```python
from build123d import *

# Parameters (mm, degrees)
ESBO_O1_W                = 170.2
ESBO_O1_H                = 111.2
RESSALTO_EXTRUS_O1_DEPTH = 0.9
ESBO_O4_W                = 176.2
ESBO_O4_H                = 117.2
RESSALTO_EXTRUS_O3_DEPTH = 1
ESBO_O5_W                = 32
ESBO_O5_H                = 1.9
CORTE_EXTRUS_O3_DEPTH    = 5
ESBO_O6_R                = 1.25
RESSALTO_EXTRUS_O4_DEPTH = 2.5
ESBO_O10_W               = 13
ESBO_O10_H               = 4
CORTE_EXTRUS_O6_DEPTH    = 1.1
ESBO_O12_W               = 146.2
ESBO_O12_H               = 82.2
CORTE_EXTRUS_O8_DEPTH    = 10


with BuildPart() as part:
    # Esboço1 → Ressalto-extrusão1 (new body)
    with BuildSketch(Plane.XY):
        with Locations((91, 62.6)):
            Rectangle(ESBO_O1_W, ESBO_O1_H)
    extrude(amount=RESSALTO_EXTRUS_O1_DEPTH)

    # Esboço4 → Ressalto-extrusão3 (add)
    with BuildSketch(Plane(origin=(0, 0, 0), x_dir=(-1, 0, 0), z_dir=(0, 0, -1))):
        with Locations((-91, 62.6)):
            Rectangle(ESBO_O4_W, ESBO_O4_H)
    extrude(amount=RESSALTO_EXTRUS_O3_DEPTH)

    # Esboço5 → Corte-extrusão3 (cut)
    with BuildSketch(Plane.XZ.offset(-4)):
        with Locations((91, -0.05)):
            Rectangle(ESBO_O5_W, ESBO_O5_H)
    extrude(amount=-CORTE_EXTRUS_O3_DEPTH, mode=Mode.SUBTRACT)

    # Esboço6 → Ressalto-extrusão4 (add)
    with BuildSketch(Plane(origin=(0, 0, -1), x_dir=(-1, 0, 0), z_dir=(0, 0, -1))):
        with Locations((-108.3, 14.75)):
            Circle(ESBO_O6_R)
        with Locations((-108.3, 106.45)):
            Circle(ESBO_O6_R)
        with Locations((-43.3, 106.45)):
            Circle(ESBO_O6_R)
        with Locations((-44, 16.15)):
            Circle(ESBO_O6_R)
    extrude(amount=RESSALTO_EXTRUS_O4_DEPTH)

    # Esboço10 → Corte-extrusão6 (cut)
    with BuildSketch(Plane(origin=(0, 0, -1), x_dir=(-1, 0, 0), z_dir=(0, 0, -1))):
        with Locations((-52.05, 106.45)):
            Rectangle(ESBO_O10_W, ESBO_O10_H)
    extrude(amount=-CORTE_EXTRUS_O6_DEPTH, mode=Mode.SUBTRACT)

    # Esboço12 → Corte-extrusão8 (cut)
    with BuildSketch(Plane.XY.offset(0.9)):
        with Locations((91, 60.1)):
            Rectangle(ESBO_O12_W, ESBO_O12_H)
    extrude(amount=-CORTE_EXTRUS_O8_DEPTH, mode=Mode.SUBTRACT)


solid = part.part
```
Read the model definition and answer for the solid it produces. Units are mm, in the model's axes. Give positions to 0.01 mm unless a question says otherwise; leave off trailing zeros. Write each loop counter-clockwise with the first axis right and the second up, starting at its lowest first coordinate (ties: lowest second). Pieces come first, ordered by that corner, then holes. Notation, with made-up numbers: (22, 39.25) -> (78, 39.25) arc R5 ccw to (78, 43.25) -> close; hole circle Ø4 at (7, 60.5). An arc over 180 degrees is marked (long way). Answer in a Markdown table with one row per item.
1) Each of these flat-tipped pins is pushed along its axis until it touches: pin 1 Ø3 at (x, y) = (161.5, 54) entering from +Z; pin 2 Ø0.7 at (x, z) = (157, 0.5) entering from -Y; pin 3 Ø2 at (x, y) = (53, 106) entering from -Z. Where does it stop, or does it pass through?
Results list:
| item | result |
|---|---|
| pin 1 | through |
| pin 2 | y = 7 |
| pin 3 | z = 0.1 |
2) Section C-C on z = -1.7 is taken. Give the vertices of the cut face in (x, y).
Results list:
| item | result |
|---|---|
| outline | circle Ø2.5 at (43.3, 106.45); circle Ø2.5 at (44, 16.15); circle Ø2.5 at (108.3, 14.75); circle Ø2.5 at (108.3, 106.45) |
3) Section B-B on y = 62 is taken. Give the vertices of the cut face in (x, z).
Results list:
| item | result |
|---|---|
| outline | (2.9, -1) -> (17.9, -1) -> (17.9, 0.9) -> (5.9, 0.9) -> (5.9, 0) -> (2.9, 0) -> close; (164.1, -1) -> (179.1, -1) -> (179.1, 0) -> (176.1, 0) -> (176.1, 0.9) -> (164.1, 0.9) -> close |
4) Straight lines are drawn through the part: line 1 (Y direction, x = 103, z = 0.3); line 2 (Y direction, x = 89, z = -0.9); line 3 (Y direction, x = 53.5, z = -0.3). For each, find the intervals that lie inside material, in ascending order. Write a range as [from, to].
Results list:
| item | result |
|---|---|
| line 1 | [9, 19], [101.2, 118.2] |
| line 2 | [9, 19], [101.2, 121.2] |
| line 3 | [4, 19], [101.2, 104.45], [108.45, 121.2] |
5) Section D-D on y = 111 is taken. Give the vertices of the cut face in (x, z), plus the area to 3 significant figures.
Results list:
| item | result |
|---|---|
| outline | (2.9, -1) -> (179.1, -1) -> (179.1, 0) -> (176.1, 0) -> (176.1, 0.9) -> (5.9, 0.9) -> (5.9, 0) -> (2.9, 0) -> close |
| area | 329 mm^2 |
6) Determine the mould class of faces 1 (the flat face through (90, 14, 0.9)), 2 (the flat face through (52, 106, 0.1)) for opening direction Y: released by +Y, released by -Y, zero draft, split by the parting line, or undercut.
Results list:
| item | result |
|---|---|
| face 1 | zero draft |
| face 2 | undercut |
7) Section A-A on x = 93 is taken. Give the vertices of the cut face in (y, z).
Results list:
| item | result |
|---|---|
| outline | (9, -1) -> (19, -1) -> (19, 0.9) -> (9, 0.9) -> close; (101.2, -1) -> (121.2, -1) -> (121.2, 0) -> (118.2, 0) -> (118.2, 0.9) -> (101.2, 0.9) -> close |
